Geometry: final body of the model. Coordinates: model frame, mm. A direction names the side the tool comes from. Give positions to 0.01 mm unless a question says otherwise; leave off trailing zeros. Order: outer loops, then holes, each group sorted by start corner. A loop starts at its lowest first (then second) coordinate and runs counter-clockwise, first axis right, second up. Notation, with made-up numbers: M -3.5,87 L 33.5,87 A37 ccw 33.5,123 Z; hole C 71,62.5 d11. An arc over 180 degrees is marked long. One line per item, written item: value. Start each with the question number.
```python
from build123d import *

# Parameters (mm, degrees)
F0_R     = 1.27
F1_DEPTH = 5.08
F2_R     = 1.905
F2_R_2   = 1.27
F3_DEPTH = 1.905
F5_DEPTH = 1.27


with BuildPart() as f1:
    # F0 (on Front) → F1 (new body)
    with BuildSketch(Plane.XZ):
        Circle(F0_R)
    extrude(amount=F1_DEPTH)

    # F2 (on face) → F3 (join)
    with BuildSketch(Plane.XZ.offset(5.08)):
        Circle(F2_R)
        Circle(F2_R_2, mode=Mode.SUBTRACT)
        Circle(F2_R_2)
    extrude(amount=F3_DEPTH)

    # F4 (on face) → F5 (cut)
    with BuildSketch(Plane.XZ.offset(6.985)):
        Polygon((1.385297, 0.832218), (-0.028074, 1.615811), (-1.413371, 0.783593), (-1.385297, -0.832218), (0.028074, -1.615811), (1.413371, -0.783593), align=None)
    extrude(amount=-F5_DEPTH, mode=Mode.SUBTRACT)


solid = f1.part
```
Q1. Section query B-B on z = -1.45. Return loops of the section in (x, y) (3 decimals), and give its area (3 significant figures).
Q2. Ray query, line 1 along Y through (x, z) = (-0.55, 1.1) (3 decimals); line 2 along X through (y, z) = (-6, -1); line 3 along Y through (x, z) = (-1.2, 1) (3 decimals). Return the intervals inside material, ascending. Write a range as [from, to].
Q3. Mould query, pull axis Z, two halves, no side actions, for faces 3 (the face through (-0.41, -6.02, -1.86)), 4 (the face through (-0.711, -6.359, 1.206)), 5 (the face through (0, 0, 0)), 6 (the face through (-0.689, -6.359, -1.219)). Classes: +Z half, -Z half, draft (parallel to the pull), parting line (faces both ways), or undercut.
Q4. Section query C-C on x = -1.05. Return loops of the section in (y, z) (1 decimal).
Q5. Set-up query: faces 1 (the face through (0.689, -6.359, 1.219)), 2 (the face through (-0.17, -2.5, 1.26)). Return all of +Z, -Z, +X, -X, +Y, -Y with unobstructed straight access to the full face (end or side cutting, diameter ignored); none if empty.
Q6. Section query A-A on y = -6. Return loops of the section in (x, z) (3 decimals).
Q7. Section query D-D on y = -1. Return loops of the section in (x, z), and give its area (3 significant figures).
Results below:
1. outline: M -1.236,-6.985 L -0.271,-6.985 L -0.271,-5.715 L 0.304,-5.715 L 0.304,-6.985 L 1.236,-6.985 L 1.236,-5.08 L -1.236,-5.08 Z
1. area: 3.98 mm2
2. line 1: [-5.715, 0]
2. line 2: [-1.62, -1.08], [1.05, 1.62]
2. line 3: [-6.985, -5.08]
3. face 3: parting line
3. face 4: undercut
3. face 5: draft
3. face 6: undercut
4. outline: M -7,-1.6 L -5.1,-1.6 L -5.1,-0.7 L 0,-0.7 L 0,0.7 L -5.1,0.7 L -5.1,1.6 L -7,1.6 L -7,1 L -5.7,1 L -5.7,-1 L -7,-1 Z
5. face 1: -Y
5. face 2: +Y
6. outline: C 0,0 d3.81; hole M -1.413,0.784 L -1.385,-0.832 L 0.028,-1.616 L 1.413,-0.784 L 1.385,0.832 L -0.028,1.616 Z
7. outline: C 0,0 d2.54
7. area: 5.07 mm2
